Source: three-view drawing plus pictorial views. Frame: mm from the lowest corner of the part. Give positions to 0.01 mm unless a question says otherwise; leave off trailing zeros. Loops run counter-clockwise (first coordinate to the right, second up) from the corner with the lowest first, then second, coordinate; pieces in that order, holes last. Notation, with made-up numbers: (44.5, 77) - (102.5, 77) arc R12 ccw to (102.5, 82) - close; hole circle Ø6 at (71, 40). An arc over 180 degrees is marked (long way). Answer as a JSON object with one key per item and string values. Group by question number.
(1) Section query D-D (x = 8.75). Return loops of the section in (y, z), plus the area to 3 significant figures.
(2) Section query A-A (z = 5). Return loops of the section in (x, y).
(3) Section query B-B (x = 5). Return loops of the section in (y, z), plus the area to 3 significant figures.
(4) Mould query, pull axis X, two halves, no side actions, for the marked faces 1, 2 and 3. Classes: +X half, -X half, draft (parallel to the pull), parting line (faces both ways), or undercut.
(5) Material intervals for L1, parallel to Z at x = 5, y = 6.75; L2, parallel to Y at x = 9.5, z = 3.75; L3, parallel to X at y = 15.25, z = 5.25, sorted ascending.
(6) Section query C-C (y = 10). Return loops of the section in (x, z), plus the area to 3 significant figures.
(7) Pin query (flat end, axial travel): P1, Ø5, axis at x = 1.5, y = 4.5, coming from the -Z side; P2, Ø1.5, axis at x = 6.5, y = 12, coming from the +Z side; P3, Ø5, axis at x = 5.5, y = 2, coming from the +Z side. Return the tip coordinate at first contact, or that it passes through.
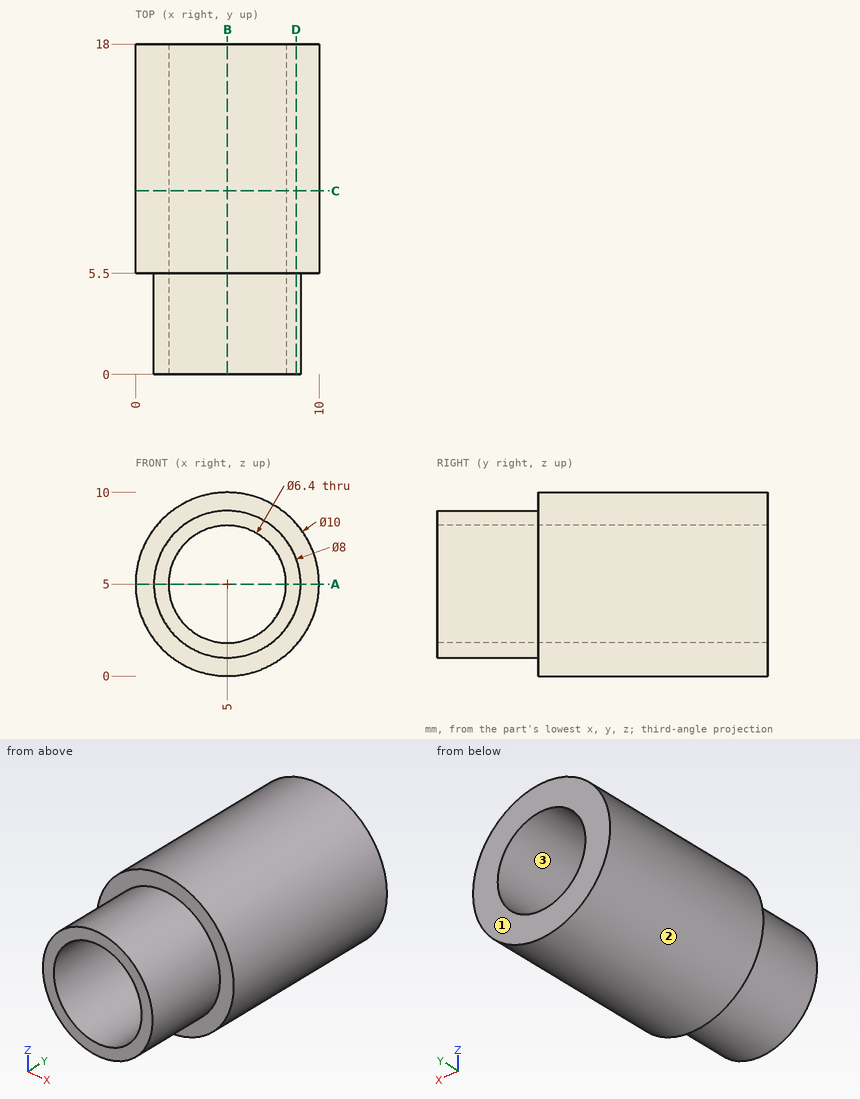
Recorded:
{
 "1": {"outline": "(0, 3.61) - (5.5, 3.61) - (5.5, 1.69) - (18, 1.69) - (18, 8.31) - (5.5, 8.31) - (5.5, 6.39) - (0, 6.39) - close", "area": "98.0 mm^2"},
 "2": {"outline": "(0, 5.5) - (1, 5.5) - (1, 0) - (1.8, 0) - (1.8, 18) - (0, 18) - close; (8.2, 0) - (9, 0) - (9, 5.5) - (10, 5.5) - (10, 18) - (8.2, 18) - close"},
 "3": {"outline": "(0, 1) - (5.5, 1) - (5.5, 0) - (18, 0) - (18, 1.8) - (0, 1.8) - close; (0, 8.2) - (18, 8.2) - (18, 10) - (5.5, 10) - (5.5, 9) - (0, 9) - close", "area": "53.8 mm^2"},
 "4": {"face 1": "draft", "face 2": "parting line", "face 3": "undercut"},
 "5": {"L1": "z = 0 to 1.8, 8.2 to 10", "L2": "y = 5.5 to 18", "L3": "x = 0.01 to 1.81, 8.19 to 9.99"},
 "6": {"outline": "circle Ø10 at (5, 5); hole circle Ø6.4 at (5, 5)", "area": "46.4 mm^2"},
 "7": {"P1": "stops at z = 0.15", "P2": "stops at z = 9.94", "P3": "stops at z = 9"}
}
